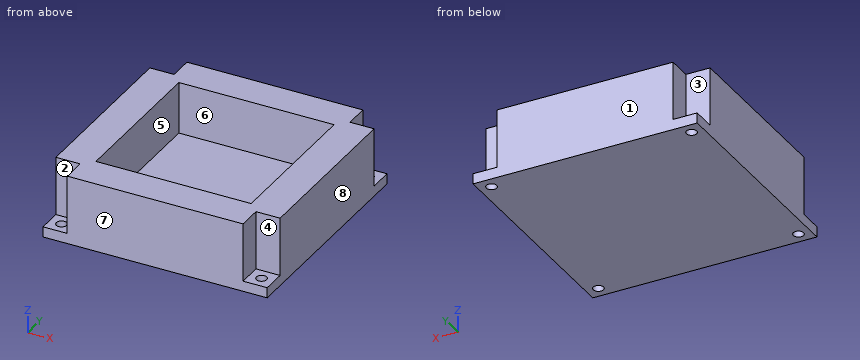
from build123d import *

# Parameters (mm, degrees)
SKETCH_1_W               = 65
SKETCH_1_H               = 65
EXTRUDE_4_DEPTH          = 20
SKETCH_3_W               = 45
SKETCH_3_H               = 45
CUT_EXTRUDE_1_DEPTH      = 15
SKETCH_4_W               = 7
SKETCH_4_H               = 7
CUT_EXTRUDE_2_DEPTH      = 17
PATTERN_CIRCULAR_1_COUNT = 4
SKETCH_5_R               = 1.5
CUT_EXTRUDE_3_DEPTH      = 3
PATTERN_CIRCULAR_2_COUNT = 4


with BuildPart() as part:
    # Эскиз1 → Бобышка-Вытянуть4 (new body)
    with BuildSketch(Plane.XY):
        Rectangle(SKETCH_1_W, SKETCH_1_H)
    extrude(amount=EXTRUDE_4_DEPTH)

    # Эскиз3 → Вырез-Вытянуть1 (cut)
    with BuildSketch(Plane.XY.offset(20)):
        Rectangle(SKETCH_3_W, SKETCH_3_H)
    extrude(amount=-CUT_EXTRUDE_1_DEPTH, mode=Mode.SUBTRACT)

    # Эскиз4 → Вырез-Вытянуть2 (cut)
    with BuildSketch(Plane.XY.offset(20)):
        with Locations((-29, 29)):
            Rectangle(SKETCH_4_W, SKETCH_4_H)
    cut_extrude_2 = extrude(amount=-CUT_EXTRUDE_2_DEPTH, mode=Mode.SUBTRACT)

    # Круговой массив1: Вырез-Вытянуть2 ×4 about axis
    pattern_circular_1_axis = Axis((0, 0, 0), (0, 0, 1))
    for i in range(1, PATTERN_CIRCULAR_1_COUNT):
        add(cut_extrude_2.rotate(pattern_circular_1_axis, i * 360 / PATTERN_CIRCULAR_1_COUNT), mode=Mode.SUBTRACT)

    # Эскиз5 → Вырез-Вытянуть3 (cut)
    with BuildSketch(Plane.XY.offset(3)):
        with Locations((-29, 29)):
            Circle(SKETCH_5_R)
    cut_extrude_3 = extrude(amount=-CUT_EXTRUDE_3_DEPTH, mode=Mode.SUBTRACT)

    # Круговой массив2: Вырез-Вытянуть3 ×4 about axis
    pattern_circular_2_axis = Axis((0, 0, 0), (0, 0, 1))
    for i in range(1, PATTERN_CIRCULAR_2_COUNT):
        add(cut_extrude_3.rotate(pattern_circular_2_axis, i * 360 / PATTERN_CIRCULAR_2_COUNT), mode=Mode.SUBTRACT)


solid = part.part
Design review of the part built by this model. Coordinates are the model's own, in mm. Face numbers are marked on the shaded views. A direction names the side the tool comes from. Coordinates: 2 decimals unless noted, no trailing zeros. Loops run counter-clockwise (first coordinate to the right, second up) from the corner with the lowest first, then second, coordinate; pieces in that order, holes last. Notation, with made-up numbers: (-18, -6.75) - (-12, -6.75) arc R15 cw to (-12, 17.25) - close; hole circle Ø1 at (35.25, 43). An arc over 180 degrees is marked (long way). Use CSV: the item, a comma, the result in double quotes. Start each with the question number.
1. To check wall thickness, follow probe 1 along Y at (x, z) = (-29, 1.7); probe 2 along X at (y, z) = (1, 9). State the ranges of each line that lie inside material, in increasing order.
2. For the marked faces 1, 2, 3, 4 and 5, list the 3-axis set-ups (+Z, -Z, +X, -X, +Y, -Y) from which the entire face can be reached by the end or side of a thin tool; tool diameter is ignored.
3. Add section A-A on x = 29. Give the boundary of the cut face in (y, z), plus the area to 3 significant figures.
4. Mouldability with a two-part tool opening along X and no side actions: class the marked faces 6, 7 and 8 as released by +X, released by -X, zero draft, split by the parting line, or undercut.
5. Add section C-C on z = 17. Give the boundary of the cut face in (x, y), plus the area to 3 significant figures.
6. Add section D-D on y = 16. Give the boundary of the cut face in (x, z).
7. Clearance check with flat-ended pins moving along their axes: pin 1 (2 mm diameter, centred on y = -27.5, z = 11.5, fed in from +X); pin 2 (2 mm diameter, centred on x = 28.5, z = 14, fed in from +Y); pin 3 (2 mm diameter, centred on x = 29.5, z = 14.5, fed in from -Y). State where each tip first meets the part, or that it passes through.
Resolved:
1,probe 1,"-32.5 to -30.5, -27.5 to 27.5, 30.5 to 32.5"
1,probe 2,"-32.5 to -22.5, 22.5 to 32.5"
2,face 1,"+Z, -Z, +X, -X, +Y"
2,face 2,"+Z, -X, -Y"
2,face 3,"+Z, -X, +Y"
2,face 4,"+Z, +X, -Y"
2,face 5,"+Z"
3,outline,"(-32.5, 0) - (-30.5, 0) - (-30.5, 3) - (-32.5, 3) - close; (-27.5, 0) - (27.5, 0) - (27.5, 3) - (25.5, 3) - (25.5, 20) - (-25.5, 20) - (-25.5, 3) - (-27.5, 3) - close; (30.5, 0) - (32.5, 0) - (32.5, 3) - (30.5, 3) - close"
3,area,"1,040 mm2"
4,face 6,"undercut"
4,face 7,"zero draft"
4,face 8,"released by +X"
5,outline,"(-32.5, -25.5) - (-25.5, -25.5) - (-25.5, -32.5) - (25.5, -32.5) - (25.5, -25.5) - (32.5, -25.5) - (32.5, 25.5) - (25.5, 25.5) - (25.5, 32.5) - (-25.5, 32.5) - (-25.5, 25.5) - (-32.5, 25.5) - close; hole (-22.5, -22.5) - (22.5, -22.5) - (22.5, 22.5) - (-22.5, 22.5) - close"
5,area,"2,000 mm2"
6,outline,"(-32.5, 0) - (32.5, 0) - (32.5, 20) - (22.5, 20) - (22.5, 5) - (-22.5, 5) - (-22.5, 20) - (-32.5, 20) - close"
7,pin 1,"x = 25.5"
7,pin 2,"y = 25.5"
7,pin 3,"y = -25.5"
